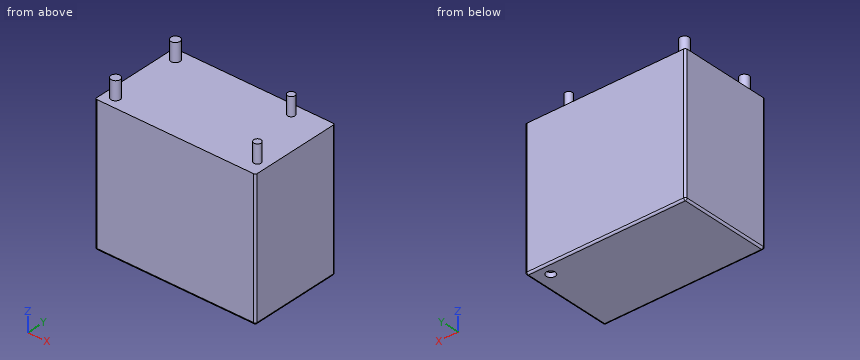
```python
from build123d import *

# Parameters (mm, degrees)
SKETCH_1_W          = 17.6
SKETCH_1_H          = 10.1
EXTRUDE_1_DEPTH     = 15
SKETCH_2_R          = 0.5
SKETCH_2_R_2        = 0.4
EXTRUDE_2_DEPTH     = 2
FILLET_1_R          = 0.2
SKETCH_3_R          = 0.5
CUT_EXTRUDE_1_DEPTH = 0.5


with BuildPart() as part:
    # 草图1 → 凸台-拉伸1 (new body)
    with BuildSketch(Plane.XY):
        with Locations((8.8, 5.05)):
            Rectangle(SKETCH_1_W, SKETCH_1_H)
    extrude(amount=-EXTRUDE_1_DEPTH)

    # 草图2 → 凸台-拉伸2 (add)
    with BuildSketch(Plane.XY):
        with Locations(Location((1.18, 8.86, 0), (0, 0, 180))):
            Circle(SKETCH_2_R)
        with Locations(Location((13.88, 8.86, 0), (0, 0, 180))):
            Circle(SKETCH_2_R_2)
        with Locations(Location((16.42, 1.606982533, 0), (0, 0, 180))):
            Circle(SKETCH_2_R_2)
        with Locations(Location((1.18, 1.24, 0), (0, 0, 180))):
            Circle(SKETCH_2_R)
    extrude(amount=EXTRUDE_2_DEPTH)

    # 圆角1
    fillet_1_edges = [part.edges().sort_by_distance(p)[0] for p in [
        (17.6, 5.05, -15),
        (8.8, 10.1, -15),
        (0, 5.05, -15),
        (8.8, 0, -15),
        (0, 10.1, -7.5),
        (17.6, 10.1, -7.5),
        (17.6, 0, -7.5),
        (0, 0, -7.5),
    ]]
    fillet(fillet_1_edges, radius=FILLET_1_R)

    # 草图3 → 切除-拉伸1 (cut)
    with BuildSketch(Plane(origin=(0, 0, -15), x_dir=(-1, 0, 0), z_dir=(0, 0, -1))):
        with Locations((-15.910317982, 8.793351903)):
            Circle(SKETCH_3_R)
    extrude(amount=-CUT_EXTRUDE_1_DEPTH, mode=Mode.SUBTRACT)


solid = part.part
```
Work out the finished part from the listing and answer in its coordinate system (mm). Give positions to 0.01 mm unless a question says otherwise; leave off trailing zeros. Loops run counter-clockwise (first coordinate to the right, second up) from the corner with the lowest first, then second, coordinate; pieces in that order, holes last. Notation, with made-up numbers: (16.5, 19) - (32.5, 19) arc R18 ccw to (32.5, 41) - close; hole circle Ø7 at (-37.75, -12.5). An arc over 180 degrees is marked (long way). Use CSV: the item, a comma, the result in double quotes. Start each with the question number.
(1) Find section B-B, the plane x = 1.18. Determine the outline of the cut face in (y, z), plus the area to 3 significant figures.
(2) Find section A-A, the plane x = 7.5. Determine the outline of the cut face in (y, z).
(3) Find section C-C, the plane x = 13.88. Determine the outline of the cut face in (y, z), plus the area to 3 significant figures.
(4) Find the intervals of material crossed by L1, parallel to Z at x = 8.75, y = 7.75; L2, parallel to Y at x = 16.75, z = 0.5, in increasing order.
(5) This flat-tipped pin is pushed along its axis until it touches: pin 1 (5 mm diameter, centred on x = 6.5, y = 4.5, fed in from +Z). Where does it stop, or does it pass through?
Results found:
1,outline,"(0, -14.8) arc R0.2 ccw to (0.2, -15) - (9.9, -15) arc R0.2 ccw to (10.1, -14.8) - (10.1, 0) - (9.36, 0) - (9.36, 2) - (8.36, 2) - (8.36, 0) - (1.74, 0) - (1.74, 2) - (0.74, 2) - (0.74, 0) - (0, 0) - close"
1,area,"155 mm^2"
2,outline,"(0, -14.8) arc R0.2 ccw to (0.2, -15) - (9.9, -15) arc R0.2 ccw to (10.1, -14.8) - (10.1, 0) - (0, 0) - close"
3,outline,"(0, -14.8) arc R0.2 ccw to (0.2, -15) - (9.9, -15) arc R0.2 ccw to (10.1, -14.8) - (10.1, 0) - (9.26, 0) - (9.26, 2) - (8.46, 2) - (8.46, 0) - (0, 0) - close"
3,area,"153 mm^2"
4,L1,"-15 to 0"
4,L2,"1.38 to 1.83"
5,pin 1,"z = 0"
